Could you check a few things on this model? Use its own coordinates, in mm. Face numbers are marked on the shaded views. A direction names the side the tool comes from. Give positions to 0.01 mm unless a question says otherwise; leave off trailing zeros. Order: outer loops, then holes, each group sorted by start corner. A loop starts at its lowest first (then second) coordinate and runs counter-clockwise, first axis right, second up.
Autodesk Inventor part; units mm, degrees
ref_plane "YZ Plane" through (0, 0, 0) normal (1, 0, 0) x (0, 1, 0)
ref_plane "XZ Plane" through (0, 0, 0) normal (0, 1, 0) x (-1, 0, 0)
ref_plane "XY Plane" through (0, 0, 0) normal (0, 0, 1) x (1, 0, 0)
sketch "Sketch1" plane through (0, 0, 0) normal (0, 0, 1) x (1, 0, 0)
  circle A0 centre (0, 0) radius 5.4991
  dimension "d0" = 10.9982
extrude "Extrusion1" add sketch "Sketch1" against normal blind 0.9906
sketch "Sketch2" plane through (0, 0, -0.9906) normal (0, 0, -1) x (-1, 0, 0)
  circle A0 centre (0, 0) radius 5.4991
  circle A1 centre (0, 0) radius 4.4958
  dimension "d3" = 8.9916
extrude "Extrusion2" add sketch "Sketch2" along normal blind 2.9972 contours A1
sketch "Sketch3" plane through (0, 0, 0) normal (0, 0, 1) x (1, 0, 0)
  circle A0 centre (0, 0) radius 5.4991
hole "Hole1" at (0, 0, 0) direction (0, 0, -1) diameter 7.0612 end through all
properties part number "276-2181-011 Rev1"
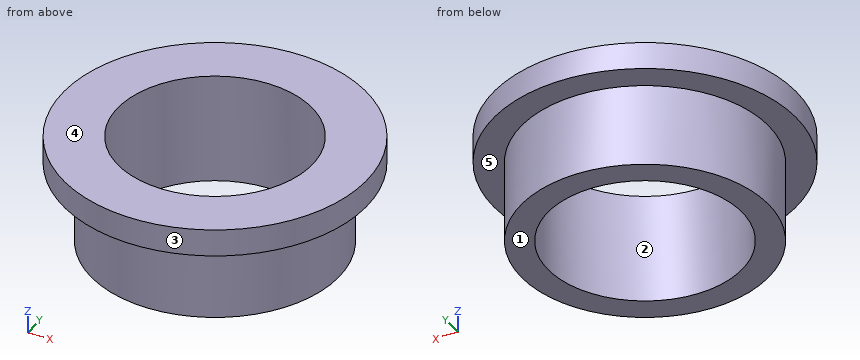
Item 1: Imagine slicing it at A-A on y = 0. List the corners of the cut face in (x, z) for me.
Findings:
outline: (-5.5, -0.99) - (-4.5, -0.99) - (-4.5, -3.99) - (-3.53, -3.99) - (-3.53, 0) - (-5.5, 0) - close; (3.53, -3.99) - (4.5, -3.99) - (4.5, -0.99) - (5.5, -0.99) - (5.5, 0) - (3.53, 0) - close
Item 2: Please list where these lines run through material, in increasing order: line 1 along Y through (x, z) = (0, -1.65); line 2 along X through (y, z) = (-0.5, -0.35); line 3 along Y through (x, z) = (1.5, -1.35).
Findings:
line 1: y = -4.5 to -3.53, 3.53 to 4.5
line 2: x = -5.48 to -3.5, 3.5 to 5.48
line 3: y = -4.24 to -3.2, 3.2 to 4.24
Item 3: For the marked faces 4 and 5, which set-ups out of +Z, -Z, +X, -X, +Y, -Y let a thin tool reach every point of the face, with its end or its side?
Findings:
face 4: +Z, +X, -X, +Y, -Y
face 5: -Z
Item 4: Imagine slicing it at C-C on z = -3.65. List the corners of the cut face in (x, y) for me.
Findings:
outline: circle Ø8.99 at (0, 0); hole circle Ø7.06 at (0, 0)
Item 5: Imagine slicing it at D-D on x = 3.75. List the corners of the cut face in (y, z) for me.
Findings:
outline: (-4.02, -0.99) - (-2.48, -0.99) - (-2.48, -3.99) - (2.48, -3.99) - (2.48, -0.99) - (4.02, -0.99) - (4.02, 0) - (-4.02, 0) - close
Item 6: We'd pull the mould along X, two halves only. Please class the marked faces 1, 2 and 3: +X half, -X half, draft (parallel to the pull), parting line (faces both ways), or undercut.
Findings:
face 1: draft
face 2: undercut
face 3: parting line
